```python
from build123d import *

# Parameters (mm, degrees)
SKETCH1_W           = 128.2
SKETCH1_H           = 16.05
BOSS_EXTRUDE1_DEPTH = 6.65
SKETCH2_R           = 1.5
SKETCH2_W           = 114
SKETCH2_H           = 2.75
CUT_EXTRUDE1_DEPTH  = 4
BOSS_EXTRUDE2_DEPTH = 0.65
BOSS_EXTRUDE3_DEPTH = 0.65


with BuildPart() as part:
    # Sketch1 → Boss-Extrude1 (new body)
    with BuildSketch(Plane(origin=(0, 0, 0), x_dir=(1, 0, 0), z_dir=(0, 1, 0))):
        Rectangle(SKETCH1_W, SKETCH1_H)
    extrude(amount=-BOSS_EXTRUDE1_DEPTH)

    # Sketch2 → Cut-Extrude1 (cut)
    with BuildSketch(Plane(origin=(0, 0, 0), x_dir=(1, 0, 0), z_dir=(0, 1, 0))):
        with Locations(Location((-60, 0, 0), (0, 0, 270))):
            Circle(SKETCH2_R)
        with Locations(Location((60, 0, 0), (0, 0, 90))):
            Circle(SKETCH2_R)
        Rectangle(SKETCH2_W, SKETCH2_H)
    extrude(amount=-CUT_EXTRUDE1_DEPTH, mode=Mode.SUBTRACT)

    # Sketch3 → Boss-Extrude2 (add)
    with BuildSketch(Plane.ZY.offset(64.09)):
        Polygon((-6.875, -6.65), (-6.875, -8.15), (-6.075, -8.15), (-6.075, -11.65), (-5.175, -11.65), (-5.175, -8.15), (-4.375, -8.15), (-4.375, -6.65), align=None)
        Polygon((-0.625, -6.65), (-3.125, -6.65), (-3.125, -8.15), (-2.325, -8.15), (-2.325, -11.65), (-1.425, -11.65), (-1.425, -8.15), (-0.625, -8.15), align=None)
        Polygon((3.125, -6.65), (0.625, -6.65), (0.625, -8.15), (1.425, -8.15), (1.425, -11.65), (2.325, -11.65), (2.325, -8.15), (3.125, -8.15), align=None)
        Polygon((6.875, -6.65), (4.375, -6.65), (4.375, -8.15), (5.175, -8.15), (5.175, -11.65), (6.075, -11.65), (6.075, -8.15), (6.875, -8.15), align=None)
    extrude(amount=-BOSS_EXTRUDE2_DEPTH)

    # Sketch4 → Boss-Extrude3 (add)
    with BuildSketch(Plane(origin=(64.09, 0, 0), x_dir=(0, 0, -1), z_dir=(1, 0, 0))):
        Polygon((-0.625, -8.15), (-0.625, -6.65), (-3.125, -6.65), (-3.125, -8.15), (-2.325, -8.15), (-2.325, -11.65), (-1.425, -11.65), (-1.425, -8.15), align=None)
        Polygon((3.125, -8.15), (3.125, -6.65), (0.625, -6.65), (0.625, -8.15), (1.425, -8.15), (1.425, -11.65), (2.325, -11.65), (2.325, -8.15), align=None)
    extrude(amount=-BOSS_EXTRUDE3_DEPTH)


solid = part.part
```
For this review, take the finished solid that the model builds, in its own axes (mm). A direction names the side the tool comes from. Round coordinates to 2 decimals unless told otherwise and drop trailing zeros. Write each loop counter-clockwise with the first axis right and the second up, starting at its lowest first coordinate (ties: lowest second). Pieces come first, ordered by that corner, then holes. Notation, with made-up numbers: (49.25, 47) - (57.25, 47) arc R27 cw to (57.25, 75) - close; hole circle Ø10 at (4.5, 75.5). An arc over 180 degrees is marked (long way). Answer as a JSON object with one key per item and string values.
1. Tool access review of faces 4 (the face through (-64.09, -9, -2)), 5 (the face through (57, -2, 0)), 6 (the face through (-63.44, -8.6, -5.6)): name each direction out of +Z, -Z, +X, -X, +Y, -Y from which nothing blocks a thin tool from reaching the whole face with its end or side.
Response values:
{"face 4": "+Z, -Z, -X, +Y, -Y", "face 5": "+Y", "face 6": "+Z, -Z, +X, -Y"}
2. We need section D-D on x = 60. Give the boundary of the cut face in (y, z) (3 decimals), then the cut area to 3 significant figures.
Response values:
{"outline": "(-6.65, -8.025) - (0, -8.025) - (0, -1.5) - (-4, -1.5) - (-4, 1.5) - (0, 1.5) - (0, 8.025) - (-6.65, 8.025) - close", "area": "94.7 mm2"}
3. We need section B-B on y = -9.5. Give the boundary of the cut face in (x, z) (3 decimals), then the cut area to 3 significant figures.
Response values:
{"outline": "(-64.09, -6.075) - (-63.44, -6.075) - (-63.44, -5.175) - (-64.09, -5.175) - close; (-64.09, -2.325) - (-63.44, -2.325) - (-63.44, -1.425) - (-64.09, -1.425) - close; (-64.09, 1.425) - (-63.44, 1.425) - (-63.44, 2.325) - (-64.09, 2.325) - close; (-64.09, 5.175) - (-63.44, 5.175) - (-63.44, 6.075) - (-64.09, 6.075) - close; (63.44, -2.325) - (64.09, -2.325) - (64.09, -1.425) - (63.44, -1.425) - close; (63.44, 1.425) - (64.09, 1.425) - (64.09, 2.325) - (63.44, 2.325) - close", "area": "3.51 mm2"}
4. To check wall thickness, follow line 1 along X through (y, z) = (-1.55, 0); line 2 along Z through (x, y) = (-31, -3.5) (3 decimals); line 3 along X through (y, z) = (-3.75, -1). State the ranges of each line that lie inside material, in increasing order.
Response values:
{"line 1": "x = -64.1 to -61.5, -58.5 to -57, 57 to 58.5, 61.5 to 64.1", "line 2": "z = -8.025 to -1.375, 1.375 to 8.025", "line 3": "x = -64.1 to -61.12, -58.88 to -57, 57 to 58.88, 61.12 to 64.1"}
5. We need section A-A on y = -1.75. Give the boundary of the cut face in (x, z) (3 decimals), then the cut area to 3 significant figures.
Response values:
{"outline": "(-64.1, -8.025) - (64.1, -8.025) - (64.1, 8.025) - (-64.1, 8.025) - close; hole circle Ø3 at (-60, 0); hole (-57, -1.375) - (57, -1.375) - (57, 1.375) - (-57, 1.375) - close; hole circle Ø3 at (60, 0)", "area": "1,730 mm2"}
6. For pin 1 Ø8 at (x, z) = (25, 2.5) entering from -Y; pin 2 Ø3 at (y, z) = (-9, 2) entering from +X; pin 3 Ø0.8 at (y, z) = (-10, -5.5) entering from -X, all flat-tipped, find the tip position at first contact; note any pin that passes through.
Response values:
{"pin 1": "stops at y = -6.65", "pin 2": "stops at x = 64.09", "pin 3": "stops at x = -64.09"}
7. Draft analysis for pull direction X (two halves, no side actions). For faces 1 (the face through (-1, -3, 8.025)), 2 (the face through (64.09, -9, -2)), 3 (the face through (-63.44, -9, -2)), state which applies: +X half, -X half, draft (parallel to the pull), parting line (faces both ways), or undercut.
Response values:
{"face 1": "draft", "face 2": "+X half", "face 3": "undercut"}
8. We need section C-C on x = -36. Give the boundary of the cut face in (y, z) (3 decimals), then the cut area to 3 significant figures.
Response values:
{"outline": "(-6.65, -8.025) - (0, -8.025) - (0, -1.375) - (-4, -1.375) - (-4, 1.375) - (0, 1.375) - (0, 8.025) - (-6.65, 8.025) - close", "area": "95.7 mm2"}
